from build123d import *

# Parameters (mm, degrees)
BOSS_EXTRUDE1_DEPTH     = 100
CUT_EXTRUDE3_DEPTH      = 554.165701555
CUT_EXTRUDE3_DEPTH_BACK = 554.165701555
CUT_EXTRUDE5_DEPTH      = 553.962044682
CUT_EXTRUDE5_DEPTH_BACK = 553.962044682
CUT_EXTRUDE7_DEPTH      = 553.962044682
CUT_EXTRUDE7_DEPTH_BACK = 553.962044682


with BuildPart() as part:
    # Sketch1 → Boss-Extrude1 (new body)
    with BuildSketch(Plane.XY):
        with BuildLine():
            ThreePointArc((-192.629438793, 0), (-136.135725272, 33.719619965), (-73.991525193, 55.321722514))
            ThreePointArc((-73.991525193, 55.321722514), (231.264395529, 54.89097703), (535.785554592, 33.719619965))
            ThreePointArc((535.785554592, 33.719619965), (536.798211586, 12.89819156), (539.317827414, -7.795017256))
            ThreePointArc((539.317827414, -7.795017256), (238.042039648, -55.533392614), (-66.568309368, -71.614065728))
            ThreePointArc((-66.568309368, -71.614065728), (-137.800866021, -50.244872094), (-192.629438793, 0))
        make_face()
    extrude(amount=BOSS_EXTRUDE1_DEPTH)

    # Sketch2 → Cut-Extrude3 (cut, two sides: drawn at the far end of the back side and taken through both)
    with BuildSketch(Plane(origin=(0, 0, 0), x_dir=(0, 0, -1), z_dir=(1, 0, 0)).offset(-CUT_EXTRUDE3_DEPTH_BACK)):
        with BuildLine():
            ThreePointArc((-65.447202994, 54.830423707), (-80.892507985, 50.983746932), (-92.956496986, 40.600368972))
            ThreePointArc((-92.956496986, 40.600368972), (-98.736407831, -10.977338679), (-88.967303886, -61.950193259))
            ThreePointArc((-88.967303886, -61.950193259), (-83.10915251, -68.165990231), (-75.589128758, -72.216090516))
            ThreePointArc((-75.589128758, -72.216090516), (-123.822815089, -94.064788666), (-173.378544397, -75.407784602))
            ThreePointArc((-173.378544397, -75.407784602), (-163.802190068, -4.583325871), (-135.262897635, 60.940099743))
            ThreePointArc((-135.262897635, 60.940099743), (-100.366866686, 80.430667917), (-61.326949176, 89.003885783))
            ThreePointArc((-61.326949176, 89.003885783), (-63.560434952, 71.938056418), (-65.447202994, 54.830423707))
        make_face()
    extrude(amount=CUT_EXTRUDE3_DEPTH + CUT_EXTRUDE3_DEPTH_BACK, mode=Mode.SUBTRACT)

    # Sketch3 → Cut-Extrude5 (cut, two sides: drawn at the far end of the back side and taken through both)
    with BuildSketch(Plane(origin=(0, 0, 0), x_dir=(0, 0, -1), z_dir=(1, 0, 0)).offset(-CUT_EXTRUDE5_DEPTH_BACK)):
        with BuildLine():
            ThreePointArc((-74.208303325, 50.886642831), (-50.335012976, 52.211638999), (-26.713093985, 48.511024166))
            ThreePointArc((-26.713093985, 48.511024166), (-16.247111553, 43.841102683), (-7.714956491, 36.189482926))
            ThreePointArc((-7.714956491, 36.189482926), (-2.445034952, -12.786836037), (-8.678058045, -61.649923489))
            ThreePointArc((-8.678058045, -61.649923489), (-17.453523943, -70.69509128), (-29.511303704, -74.360307413))
            ThreePointArc((-29.511303704, -74.360307413), (33.955140221, -79.826327987), (85.286434054, -42.104117568))
            ThreePointArc((85.286434054, -42.104117568), (41.180066923, 16.064388488), (12.319514625, 83.116720583))
            ThreePointArc((12.319514625, 83.116720583), (-170.558095104, 441.821406771), (-74.208303325, 50.886642831))
        make_face()
    extrude(amount=CUT_EXTRUDE5_DEPTH + CUT_EXTRUDE5_DEPTH_BACK, mode=Mode.SUBTRACT)

    # Sketch4 → Cut-Extrude7 (cut, two sides: drawn at the far end of the back side and taken through both)
    with BuildSketch(Plane.XY.offset(-CUT_EXTRUDE7_DEPTH_BACK)):
        Polygon((-79.201401397, 32.882000093), (-79.201401397, -3.122719846), (-222.768125928, 1.814195624), (-233.222282556, 17.110218535), (-80.529357675, 72.456896947), align=None)
    extrude(amount=CUT_EXTRUDE7_DEPTH + CUT_EXTRUDE7_DEPTH_BACK, mode=Mode.SUBTRACT)


solid = part.part
Design review of the part built by this model. Coordinates are the model's own, in mm. Coordinates: 2 decimals unless noted, no trailing zeros. Loops run counter-clockwise (first coordinate to the right, second up) from the corner with the lowest first, then second, coordinate; pieces in that order, holes last. Notation, with made-up numbers: (57.5, 83.25) -> (80.5, 83.25) arc R18 cw to (80.5, 97.25) -> close; hole circle Ø4 at (81, 13). An arc over 180 degrees is marked (long way). Use a Markdown table: item, result. Add a question column.
Item 1: We need section A-A, the plane x = 1.5. Write out the cut boundary in (y, z), and give its area (3 significant figures).
Item 2: The part is to be moulded in two halves that separate along Y. For faces 1 (the flat face through (-79.201, 15, 50)), 2 (the cylindrical face through (242.291, -55.083, 49.9)), 3 (the cylindrical face through (168.22, -12.1, 2.44)), 4 (the cylindrical face through (136.738, 52.228, 50.67)), say which applies: +Y half, -Y half, draft (parallel to the pull), parting line (faces both ways), or undercut.
Item 3: We need section C-C, the plane y = -22.5. Write out the cut boundary in (x, z).
Item 4: We need section B-B, the plane z = 55.5. Write out the cut boundary in (x, y), and give its area (3 significant figures).
Item 5: Wall thickness on L1, parallel to Z at x = -117, y = -11; L2, parallel to Y at x = 159, z = 84; L3, parallel to Y at x = 413, z = 29: over which ranges is each line inside the solid? List them lowest first. Write a range as from..to.
Item 6: We need section D-D, the plane x = 253.5. Write out the cut boundary in (y, z).
Item 7: Clearance check with flat-ended pins moving along their axes: P1, Ø1, axis at x = 180, z = 50, coming from the -Y side; P2, Ø3, axis at y = 16, z = 42, coming from the +X side; P3, Ø1.5, axis at x = 203, z = 52, coming from the -Y side. State where each tip first meets the part, or that it passes through.
Numbers:
| question | item | result |
|---|---|---|
| 1 | outline | (-70.78, 17.6) arc R25.2 ccw to (-61.65, 8.68) arc R210.93 ccw to (36.19, 7.71) arc R36.96 ccw to (48.51, 26.71) arc R113.61 ccw to (50.89, 74.21) arc R202.65 cw to (49.99, 82.69) arc R34.43 ccw to (40.6, 92.96) arc R173.11 ccw to (-61.95, 88.97) arc R26.72 ccw to (-70.78, 78.96) -> close |
| 1 | area | 10,700 mm^2 |
| 2 | face 1 | undercut |
| 2 | face 2 | -Y half |
| 2 | face 3 | parting line |
| 2 | face 4 | +Y half |
| 3 | outline | (-174, 2.76) -> (465.43, 2.76) -> (465.43, 97.9) -> (-174, 97.9) -> close |
| 4 | outline | (-192.63, 0) arc R166.54 ccw to (-66.57, -71.61) arc R2922.96 ccw to (539.32, -7.8) arc R287.33 cw to (535.79, 33.72) arc R4489.88 ccw to (291.49, 52.35) -> (-79.85, 52.35) -> (-79.2, 32.88) -> (-79.2, -3.12) -> (-191.63, 0.74) arc R323.75 ccw to start |
| 4 | area | 66,800 mm^2 |
| 5 | L1 | z = 2.44..98.74 |
| 5 | L2 | y = -62.78..49.16 |
| 5 | L3 | y = -31.74..44.76 |
| 6 | outline | (-53.86, 6.9) arc R210.93 ccw to (36.19, 7.71) arc R36.96 ccw to (48.51, 26.71) arc R113.61 ccw to (50.89, 74.21) arc R202.65 cw to (49.99, 82.69) arc R34.43 ccw to (40.6, 92.96) arc R173.11 ccw to (-53.86, 91.6) -> close |
| 7 | P1 | stops at y = -61.1 |
| 7 | P2 | stops at x = 536.67 |
| 7 | P3 | stops at y = -59.08 |
